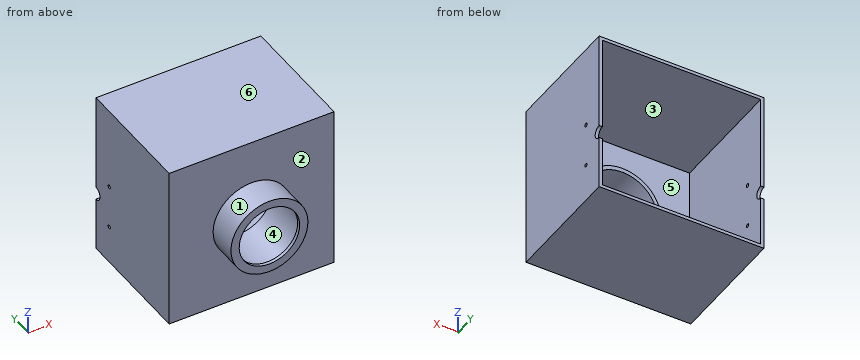
from build123d import *

# Parameters (mm, degrees)
SKETCH_1_W          = 150
SKETCH_1_H          = 150
EXTRUDE_1_DEPTH     = 3
SKETCH_2_W          = 150
SKETCH_2_H          = 150
SKETCH_2_W_2        = 144
SKETCH_2_H_2        = 144
EXTRUDE_2_DEPTH     = 107.65
SKETCH_3_R          = 31.25
CUT_EXTRUDE_1_DEPTH = 91
SKETCH_4_R          = 6
CUT_EXTRUDE_2_DEPTH = 201.9189451
SKETCH_8_R          = 35
SKETCH_8_R_2        = 31.25
EXTRUDE_4_DEPTH     = 18
SKETCH_9_R          = 1.65
CUT_EXTRUDE_3_DEPTH = 201.9189451
EXTRUDE_START       = 27
SKETCH_14_R         = 35
SKETCH_14_R_2       = 31.25
EXTRUDE_7_DEPTH     = 27
SKETCH_15_R         = 31.25
SKETCH_15_R_2       = 27.5
EXTRUDE_8_DEPTH     = 3


with BuildPart() as part:
    # 草图1 → 凸台-拉伸1 (new body)
    with BuildSketch(Plane(origin=(0, 0, 0), x_dir=(1, 0, 0), z_dir=(0, 1, 0))):
        Rectangle(SKETCH_1_W, SKETCH_1_H)
    extrude(amount=EXTRUDE_1_DEPTH)

    # 草图2 → 凸台-拉伸2 (add)
    with BuildSketch(Plane(origin=(0, 3, 0), x_dir=(1, 0, 0), z_dir=(0, 1, 0))):
        Rectangle(SKETCH_2_W, SKETCH_2_H)
        Rectangle(SKETCH_2_W_2, SKETCH_2_H_2, mode=Mode.SUBTRACT)
    extrude(amount=EXTRUDE_2_DEPTH)

    # 草图3 → 切除-拉伸1 (cut)
    with BuildSketch(Plane.XZ):
        with Locations(Location((0, 0, 0), (0, 0, 270))):
            Circle(SKETCH_3_R)
    extrude(amount=-CUT_EXTRUDE_1_DEPTH, mode=Mode.SUBTRACT)

    # 草图4 → 切除-拉伸2 (cut, through all)
    with BuildSketch(Plane.ZY.offset(75)):
        with Locations((-20.1, 110.65)):
            Circle(SKETCH_4_R)
    extrude(amount=-CUT_EXTRUDE_2_DEPTH, mode=Mode.SUBTRACT)

    # 草图8 → 凸台-拉伸4 (add)
    with BuildSketch(Plane(origin=(0, 3, 0), x_dir=(1, 0, 0), z_dir=(0, 1, 0))):
        with Locations(Location((0, 0, 0), (0, 0, 270))):
            Circle(SKETCH_8_R)
        with Locations(Location((0, 0, 0), (0, 0, 90))):
            Circle(SKETCH_8_R_2, mode=Mode.SUBTRACT)
    extrude(amount=EXTRUDE_4_DEPTH)

    # 草图9 → 切除-拉伸3 (cut, through all)
    with BuildSketch(Plane.ZY.offset(75)):
        with Locations((-40.1, 90.65)):
            Circle(SKETCH_9_R)
        with Locations((-0.1, 90.65)):
            Circle(SKETCH_9_R)
    extrude(amount=-CUT_EXTRUDE_3_DEPTH, mode=Mode.SUBTRACT)

    # 草图14 → 凸台-拉伸7 (add)
    with BuildSketch(Plane.XZ.offset(EXTRUDE_START)):
        with Locations(Location((0, 0, 0), (0, 0, 90))):
            Circle(SKETCH_14_R)
        with Locations(Location((0, 0, 0), (0, 0, 270))):
            Circle(SKETCH_14_R_2, mode=Mode.SUBTRACT)
    extrude(amount=-EXTRUDE_7_DEPTH)

    # 草图15 → 凸台-拉伸8 (add)
    with BuildSketch(Plane.XZ.offset(27)):
        with Locations(Location((0, 0, 0), (0, 0, 270))):
            Circle(SKETCH_15_R)
        with Locations(Location((0, 0, 0), (0, 0, 270))):
            Circle(SKETCH_15_R_2, mode=Mode.SUBTRACT)
    extrude(amount=-EXTRUDE_8_DEPTH)


solid = part.part
Model file for the job. Use its own axes, mm. Face numbers are marked on the shaded views. A direction names the side the tool comes from. Coordinates: 2 decimals unless noted, no trailing zeros. Loops run counter-clockwise (first coordinate to the right, second up) from the corner with the lowest first, then second, coordinate; pieces in that order, holes last. Notation, with made-up numbers: (62.25, 78.25) -> (102.25, 78.25) arc R20 cw to (102.25, 101.25) -> close; hole circle Ø3 at (81, -17.75). An arc over 180 degrees is marked (long way). Use one line per item in the form item = value. Start each with the question number.
(1) Flat gauge pins, fed straight in: pin 1 (8 mm diameter, centred on x = 42, z = 12, fed in from -Y); pin 2 (4.5 mm diameter, centred on y = 90.65, z = -0.1, fed in from +X); pin 3 (2 mm diameter, centred on y = -6, z = 29.5, fed in from +X); pin 4 (12 mm diameter, centred on x = 37.5, z = 45.5, fed in from +Y). Where does each tip first touch, or does it go through?
(2) Probe probe 1 along Z at (x, y) = (-74.35, 90.65); probe 2 along Z at (x, y) = (-34, 55); probe 3 along Y at (x, z) = (73.4, -40.1). List the from-to ranges inside material, lowest first. Write a range as from..to.
(3) Cut at D-D on x = -43. Give the cut face in (y, z).
(4) Pull direction X, two halves, no side cores. Call the marked faces 1, 2, 3 and 4: pulls with the +X half, pulls with the -X half, needs draft (parallel to the pull), parting line crosses it, or undercut.
(5) Cut at C-C on z = -20.1. Give the cut face in (x, y), and give its area (3 significant figures).
(6) Cut at A-A on x = 0. Give the cut face in (y, z).
(7) Tool access for the marked faces 5 and 6: list every direction of +Z, -Z, +X, -X, +Y, -Y with a clear straight run to the whole face (end or side of a thin tool).
(8) Cut at B-B on y = 76.5. Give the cut face in (x, z).
Values:
q1.pin_1 = 0
q1.pin_2 = 75
q1.pin_3 = 20.32
q1.pin_4 = 3
q2.probe_1 = -75..-41.75, -38.45..-1.75, 1.55..75
q2.probe_2 = -75..-72, 72..75
q2.probe_3 = 0..89, 92.3..110.65
q3.outline = (0, -75) -> (110.65, -75) -> (110.65, -72) -> (3, -72) -> (3, 72) -> (110.65, 72) -> (110.65, 75) -> (0, 75) -> close
q4.face_1 = parting line crosses it
q4.face_2 = needs draft
q4.face_3 = undercut
q4.face_4 = undercut
q5.outline = (-75, 0) -> (-28.65, 0) -> (-28.65, -27) -> (-18.77, -27) -> (-18.77, -24) -> (-23.93, -24) -> (-23.93, 21) -> (-28.65, 21) -> (-28.65, 3) -> (-72, 3) -> (-72, 104.65) -> (-75, 104.65) -> close; (18.77, -27) -> (28.65, -27) -> (28.65, 0) -> (75, 0) -> (75, 104.65) -> (72, 104.65) -> (72, 3) -> (28.65, 3) -> (28.65, 21) -> (23.93, 21) -> (23.93, -24) -> (18.77, -24) -> close
q5.area = 1,370 mm2
q6.outline = (-27, -35) -> (0, -35) -> (0, -75) -> (110.65, -75) -> (110.65, -72) -> (3, -72) -> (3, -35) -> (21, -35) -> (21, -31.25) -> (-24, -31.25) -> (-24, -27.5) -> (-27, -27.5) -> close; (-27, 27.5) -> (-24, 27.5) -> (-24, 31.25) -> (21, 31.25) -> (21, 35) -> (3, 35) -> (3, 72) -> (110.65, 72) -> (110.65, 75) -> (0, 75) -> (0, 35) -> (-27, 35) -> close
q7.face_5 = +Y
q7.face_6 = +Z, +X, -X, +Y, -Y
q8.outline = (-75, -75) -> (75, -75) -> (75, 75) -> (-75, 75) -> close; hole (-72, -72) -> (72, -72) -> (72, 72) -> (-72, 72) -> close
